Part model, mm, in its own coordinate system. Face numbers are marked on the shaded views. Coordinates: 2 decimals unless noted, no trailing zeros. Loops run counter-clockwise (first coordinate to the right, second up) from the corner with the lowest first, then second, coordinate; pieces in that order, holes last. Notation, with made-up numbers: (73.5, -37.5) - (125.5, -37.5) arc R36 cw to (125.5, -2.5) - close; hole circle Ø2 at (38.25, -35). An arc over 180 degrees is marked (long way). Use a Markdown table: item, result. Add a question column.
1. Wall check: probe 1 along X at (y, z) = (9, -99); probe 2 along Y at (x, z) = (21.4, -125); probe 3 along Y at (x, z) = (249, -81). Give the ranges that are in metal, low to high. Write a range as [from, to].
2. Drop flat-ended pins along their axis: pin 1 (5.5 mm diameter, centred on x = 23.5, y = 15, fed in from +Z); pin 2 (1.5 mm diameter, centred on x = 250, z = -103.5, fed in from +Y); pin 3 (14.5 mm diameter, centred on y = 41, z = -86, fed in from +X). Give the stop position or say it passes through.
3. Band-saw the part on B-B, the plane z = -70.5. Give the cut face in (x, y).
4. Band-saw the part on A-A, the plane x = 164.5. Give the cut face in (y, z), plus the area to 3 significant figures.
5. Band-saw the part on C-C, the plane z = -225. Give the cut face in (x, y).
6. Pull direction X, two halves, no side cores. Call the marked faces 1, 2 and 3: pulls with the +X half, pulls with the -X half, needs draft (parallel to the pull), parting line crosses it, or undercut.
from build123d import *

# Parameters (mm, degrees)
SKETCH_1_W          = 490
SKETCH_1_H          = 250
EXTRUDE_1_DEPTH     = 2
SKETCH_2_W          = 5
SKETCH_2_H          = 40
EXTRUDE_2_DEPTH     = 40
CUT_EXTRUDE_1_DEPTH = 40
SKETCH_4_R          = 10
CUT_EXTRUDE_2_DEPTH = 40
SKETCH_5_W          = 3
SKETCH_5_H          = 60
EXTRUDE_3_DEPTH     = 60
CUT_EXTRUDE_3_REACH = 359.69
SKETCH_6_R          = 25
CUT_EXTRUDE_4_REACH = 359.69
SKETCH_7_R          = 2.25
SKETCH_9_W          = 3
SKETCH_9_H          = 48.07
EXTRUDE_4_DEPTH     = 60
SKETCH_10_W         = 127.84
SKETCH_10_H         = 48.07
EXTRUDE_5_DEPTH     = 2


with BuildPart() as part:
    # 草图1 → 凸台-拉伸1 (new body)
    with BuildSketch(Plane(origin=(0, 0, 0), x_dir=(1, 0, 0), z_dir=(0, 1, 0))):
        with Locations((245, 125)):
            Rectangle(SKETCH_1_W, SKETCH_1_H)
    extrude(amount=EXTRUDE_1_DEPTH)

    # 草图2 → 凸台-拉伸2 (add)
    with BuildSketch(Plane(origin=(0, 2, 0), x_dir=(1, 0, 0), z_dir=(0, 1, 0))):
        with Locations((467.5, 125)):
            Rectangle(SKETCH_2_W, SKETCH_2_H)
    extrude_2 = extrude(amount=EXTRUDE_2_DEPTH)

    # 草图3 → 切除-拉伸1 (cut)
    with BuildSketch(Plane(origin=(470, 0, 0), x_dir=(0, 0, -1), z_dir=(1, 0, 0))):
        with BuildLine():
            ThreePointArc((105, 22), (110.857864376, 36.142135624), (125, 42))
            Line((125, 42), (105, 42))
            Line((105, 42), (105, 22))
        make_face()
        with BuildLine():
            Line((145, 42), (125, 42))
            ThreePointArc((125, 42), (139.142135624, 36.142135624), (145, 22))
            Line((145, 22), (145, 42))
        make_face()
    cut_extrude_1 = extrude(amount=-CUT_EXTRUDE_1_DEPTH, mode=Mode.SUBTRACT)

    # 草图4 → 切除-拉伸2 (cut)
    with BuildSketch(Plane(origin=(470, 0, 0), x_dir=(0, 0, -1), z_dir=(1, 0, 0))):
        with Locations((125, 22)):
            Circle(SKETCH_4_R)
    cut_extrude_2 = extrude(amount=-CUT_EXTRUDE_2_DEPTH, mode=Mode.SUBTRACT)

    # 镜向1: 凸台-拉伸2, 切除-拉伸1, 切除-拉伸2 across plane
    add(extrude_2.mirror(Plane(origin=(245, 0, 0), x_dir=(0, 0, 1), z_dir=(1, 0, 0))))
    add(cut_extrude_1.mirror(Plane(origin=(245, 0, 0), x_dir=(0, 0, 1), z_dir=(1, 0, 0))), mode=Mode.SUBTRACT)
    add(cut_extrude_2.mirror(Plane(origin=(245, 0, 0), x_dir=(0, 0, 1), z_dir=(1, 0, 0))), mode=Mode.SUBTRACT)

    # 草图5 → 凸台-拉伸3 (add)
    with BuildSketch(Plane(origin=(0, 2, 0), x_dir=(1, 0, 0), z_dir=(0, 1, 0))):
        with Locations((249.69, 81.93)):
            Rectangle(SKETCH_5_W, SKETCH_5_H)
    extrude(amount=EXTRUDE_3_DEPTH)

    # 草图6 → 切除-拉伸3 (cut, up to next)
    with BuildSketch(Plane.ZY.offset(-248.19), mode=Mode.PRIVATE) as cut_extrude_3_sk1:
        with Locations((-81.93, 32)):
            Circle(SKETCH_6_R)
    cut_extrude_3_tool1 = extrude(cut_extrude_3_sk1.sketch, amount=-CUT_EXTRUDE_3_REACH, mode=Mode.PRIVATE) & part.part
    add(cut_extrude_3_tool1.solids().sort_by_distance((248.19, 32, -81.93))[0], mode=Mode.SUBTRACT)

    # 草图7 → 切除-拉伸4 (cut, up to next)
    with BuildSketch(Plane.ZY.offset(-248.19), mode=Mode.PRIVATE) as cut_extrude_4_sk1:
        with Locations((-57.43, 56.5)):
            Circle(SKETCH_7_R)
    cut_extrude_4_tool1 = extrude(cut_extrude_4_sk1.sketch, amount=-CUT_EXTRUDE_4_REACH, mode=Mode.PRIVATE) & part.part
    # 草图7 → 切除-拉伸4 (cut, up to next)
    with BuildSketch(Plane.ZY.offset(-248.19), mode=Mode.PRIVATE) as cut_extrude_4_sk2:
        with Locations((-57.43, 7.5)):
            Circle(SKETCH_7_R)
    cut_extrude_4_tool2 = extrude(cut_extrude_4_sk2.sketch, amount=-CUT_EXTRUDE_4_REACH, mode=Mode.PRIVATE) & part.part
    # 草图7 → 切除-拉伸4 (cut, up to next)
    with BuildSketch(Plane.ZY.offset(-248.19), mode=Mode.PRIVATE) as cut_extrude_4_sk3:
        with Locations((-106.43, 7.5)):
            Circle(SKETCH_7_R)
    cut_extrude_4_tool3 = extrude(cut_extrude_4_sk3.sketch, amount=-CUT_EXTRUDE_4_REACH, mode=Mode.PRIVATE) & part.part
    # 草图7 → 切除-拉伸4 (cut, up to next)
    with BuildSketch(Plane.ZY.offset(-248.19), mode=Mode.PRIVATE) as cut_extrude_4_sk4:
        with Locations((-106.43, 56.5)):
            Circle(SKETCH_7_R)
    cut_extrude_4_tool4 = extrude(cut_extrude_4_sk4.sketch, amount=-CUT_EXTRUDE_4_REACH, mode=Mode.PRIVATE) & part.part
    add(cut_extrude_4_tool1.solids().sort_by_distance((248.19, 56.5, -57.43))[0], mode=Mode.SUBTRACT)
    add(cut_extrude_4_tool2.solids().sort_by_distance((248.19, 7.5, -57.43))[0], mode=Mode.SUBTRACT)
    add(cut_extrude_4_tool3.solids().sort_by_distance((248.19, 7.5, -106.43))[0], mode=Mode.SUBTRACT)
    add(cut_extrude_4_tool4.solids().sort_by_distance((248.19, 56.5, -106.43))[0], mode=Mode.SUBTRACT)

    # 草图9 → 凸台-拉伸4 (add)
    with BuildSketch(Plane(origin=(0, 2, 0), x_dir=(1, 0, 0), z_dir=(0, 1, 0))):
        with Locations((124.85, 75.965)):
            Rectangle(SKETCH_9_W, SKETCH_9_H)
    extrude(amount=EXTRUDE_4_DEPTH)

    # 草图10 → 凸台-拉伸5 (add)
    with BuildSketch(Plane(origin=(0, 62, 0), x_dir=(1, 0, 0), z_dir=(0, 1, 0))):
        with Locations((187.27, 75.965)):
            Rectangle(SKETCH_10_W, SKETCH_10_H)
    extrude(amount=EXTRUDE_5_DEPTH)


solid = part.part
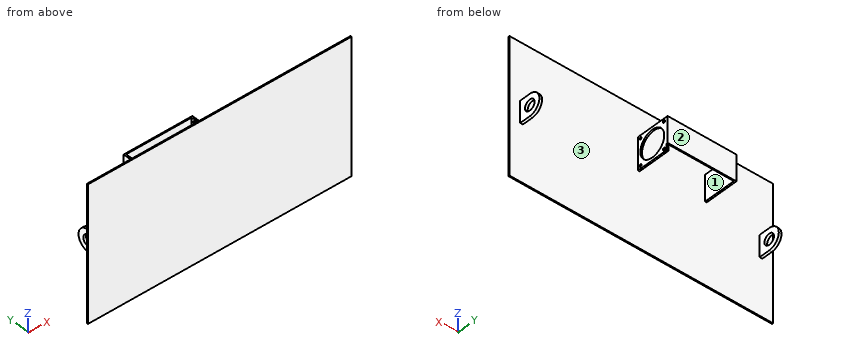
Geometry check:
| question | item | result |
|---|---|---|
| 1 | probe 1 | x = [123.35, 126.35], [248.19, 251.19] |
| 1 | probe 2 | y = [0, 12], [32, 42] |
| 1 | probe 3 | y = [0, 7.02], [56.98, 64] |
| 2 | pin 1 | stops at z = -105 |
| 2 | pin 2 | stops at y = 62 |
| 2 | pin 3 | stops at x = 126.35 |
| 3 | outline | (0, 0) - (490, 0) - (490, 2) - (251.19, 2) - (251.19, 9.77) - (248.19, 9.77) - (248.19, 2) - (126.35, 2) - (126.35, 62) - (248.19, 62) - (248.19, 54.23) - (251.19, 54.23) - (251.19, 64) - (123.35, 64) - (123.35, 2) - (0, 2) - close |
| 4 | outline | (0, -250) - (2, -250) - (2, 0) - (0, 0) - close; (62, -100) - (64, -100) - (64, -51.93) - (62, -51.93) - close |
| 4 | area | 596 mm^2 |
| 5 | outline | (0, 0) - (490, 0) - (490, 2) - (0, 2) - close |
| 6 | face 1 | undercut |
| 6 | face 2 | needs draft |
| 6 | face 3 | undercut |
